Can you work these out from the model? Positions are in its coordinate system, mm. A direction names the side the tool comes from. Round coordinates to 2 decimals unless told otherwise and drop trailing zeros. Loops run counter-clockwise (first coordinate to the right, second up) from the corner with the lowest first, then second, coordinate; pieces in that order, holes last.
from build123d import *

# Parameters (mm, degrees)
F0_R     = 15
F1_DEPTH = 40
F2_R     = 20
F4_DEPTH = 20
F5_R     = 5
F6_DEPTH = 60.001
F8_DEPTH = 60.001
F9_R     = 1.5
F11_SIZE = 1


with BuildPart() as f1:
    # F0 (on Top) → F1 (new body)
    with BuildSketch(Plane.XY):
        Circle(F0_R)
    extrude(amount=F1_DEPTH)

    # F2 (on face) → F4 (join, through all)
    with BuildSketch(Plane.XY.offset(40)):
        Circle(F2_R)
    extrude(amount=F4_DEPTH)

    # F5 (on face) → F6 (cut, through all)
    with BuildSketch(Plane.XY.offset(60)):
        Circle(F5_R)
    extrude(amount=-F6_DEPTH, mode=Mode.SUBTRACT)

    # F7 (on face) → F8 (cut, through all)
    with BuildSketch(Plane.XY.offset(60)):
        with BuildLine():
            Line((-18, -8.7177978871), (-18, 0))
            Line((-18, 0), (-18, 8.7177978871))
            ThreePointArc((-18, 8.7177978871), (-20, 0), (-18, -8.7177978871))
        make_face()
        with BuildLine():
            Line((18, 8.7177978871), (18, 0))
            Line((18, 0), (18, -8.7177978871))
            ThreePointArc((18, -8.7177978871), (19.4935886896, -4.472135955), (20, 0))
            ThreePointArc((20, 0), (19.4935886896, 4.472135955), (18, 8.7177978871))
        make_face()
    extrude(amount=-F8_DEPTH, mode=Mode.SUBTRACT)

    # F9 (on Right) → F10 (revolve, cut)
    with BuildSketch(Plane.YZ):
        with Locations((-15, 11.5)):
            Circle(F9_R)
    revolve(axis=Axis((0, 0, 0), (0, 0, -1)), mode=Mode.SUBTRACT)

    # F11
    f11_edges = [f1.edges().sort_by_distance(p)[0] for p in [
        (-15, 0, 0),
    ]]
    chamfer(f11_edges, length=F11_SIZE)


solid = f1.part
(1) If we mould it in two halves opening along X, with no side actions, what happens to faces 3 (the flat face through (-4, -4, 60)), 4 (the cylindrical face through (0, -20, 50)), 5 (the cylindrical face through (-1.08, -4.88, 30.42))? For each: released by +X, released by -X, zero draft, split by the parting line, or undercut.
Worked answers:
face 3: zero draft
face 4: split by the parting line
face 5: undercut
(2) If we section it at A-A, the plane x = 0: List the corners of the cut face in (y, z) for me, then the cut area to 3 significant figures.
Worked answers:
outline: (-20, 40) - (-15, 40) - (-15, 13) arc R1.5 cw to (-15, 10) - (-15, 1) - (-14, 0) - (-5, 0) - (-5, 60) - (-20, 60) - close; (5, 0) - (14, 0) - (15, 1) - (15, 10) arc R1.5 cw to (15, 13) - (15, 40) - (20, 40) - (20, 60) - (5, 60) - close
area: 1,390 mm2
(3) If I drill on line 1 (Y direction, x = 0, z = 39.5); line 2 (Z direction, x = -16, y = -5); line 3 (Z direction, x = 0.5, y = -14), over which ranges is the centre line in solid material (lowest first)?
Worked answers:
line 1: y = -15 to -5, 5 to 15
line 2: z = 40 to 60
line 3: z = 0.01 to 10.37, 12.63 to 60
(4) If we section it at B-B, the plane y = 0: List the corners of the cut face in (x, z) for me, then the cut area to 3 significant figures.
Worked answers:
outline: (-18, 40) - (-15, 40) - (-15, 13) arc R1.5 cw to (-15, 10) - (-15, 1) - (-14, 0) - (-5, 0) - (-5, 60) - (-18, 60) - close; (5, 0) - (14, 0) - (15, 1) - (15, 10) arc R1.5 cw to (15, 13) - (15, 40) - (18, 40) - (18, 60) - (5, 60) - close
area: 1,310 mm2
(5) If we section it at D-D, the plane z = 25: List the corners of the cut face in (x, y) for me, then the cut area to 3 significant figures.
Worked answers:
outline: circle Ø30 at (0, 0); hole circle Ø10 at (0, 0)
area: 628 mm2
(6) Will these pins go through, and if not, where does the flat tip stop? P1, Ø6, axis at x = -12.5, z = 30, coming from the +Y side; P2, Ø9, axis at x = 0, y = 0, coming from the +Z side; P3, Ø6, axis at y = 16, z = 36, coming from the +X side; P4, Ø1, axis at y = 13.5, z = 7.5, coming from the -X side.
Worked answers:
P1: stops at y = 11.61
P2: passes through
P3: stops at x = 7.48
P4: stops at x = -7.48
(7) For faces 1 (the cylindrical face through (0, 20, 50)), 2 (the cylindrical face through (-14.985, 0.66, 5.437)), which set-ups out of +Z, -Z, +X, -X, +Y, -Y let a thin tool reach every point of the face, with its end or its side?
Worked answers:
face 1: +Z, -Z, +Y
face 2: -Z
(8) If we section it at C-C, the plane z = 48: List the corners of the cut face in (x, y) for me.
Worked answers:
outline: (-18, -8.72) arc R20 ccw to (18, -8.72) - (18, 8.72) arc R20 ccw to (-18, 8.72) - close; hole circle Ø10 at (0, 0)
